Autodesk Inventor part; units mm, degrees
ref_plane "YZ Plane" through (0, 0, 0) normal (1, 0, 0) x (0, 1, 0)
ref_plane "XZ Plane" through (0, 0, 0) normal (0, 1, 0) x (-1, 0, 0)
ref_plane "XY Plane" through (0, 0, 0) normal (0, 0, 1) x (1, 0, 0)
sketch "Sketch1" plane through (0, 0, 0) normal (0, 1, 0) x (-1, 0, 0)
  circle A0 centre (0, 0) radius 10.16
  dimension "d0" = 20.32
extrude "Extrusion1" add sketch "Sketch1" along normal blind 31.75
sketch "Sketch2" plane through (0, 31.75, 0) normal (0, 1, 0) x (1, 0, 0)
  point P0 (0, 0)
  point P1 (0, 0)
hole "Hole1" at (0, 31.75, 0) direction (0, -1, 0) diameter 6.604 depth 19.05 tip angle 118
fillet "Fillet1" radius 3.175 1 edges at (10.16, 0, 0)
properties part number "legs"
Here's how the part is built. I have some questions about the finished solid (model axes, mm). Coordinates: 2 decimals unless noted, no trailing zeros. Order: outer loops, then holes, each group sorted by start corner. A loop starts at its lowest first (then second) coordinate and runs counter-clockwise, first axis right, second up. Notation, with made-up numbers: (-35, -24.75) - (-14, -24.75) arc R8 cw to (-14, -11.75) - close; hole circle Ø2 at (89.25, -33). An arc over 180 degrees is marked (long way). One line per question, with ' | ' between items. Start each with the question number.
1. I'm going to push flat-ended pins straight in: pin 1 Ø6 at (x, z) = (-5.5, 2) entering from -Y; pin 2 Ø2 at (x, y) = (-2.5, 15) entering from +Z; pin 3 Ø1.5 at (x, y) = (6, 21.5) entering from +Z; pin 4 Ø6 at (x, y) = (7, 21.5) entering from -Z. Where does each tip first touch, or does it pass through?
2. If we section it at A-A (y = 28): Write out the boundary of the cut face in (x, z), and give its area (3 significant figures).
3. If we mould it in two halves opening along Z, with no side actions, what happens to faces 1 (the cylindrical face through (1.323, 17.262, -10.074)), 2 (the cylindrical face through (1.26, 22.09, 3.05)), 3 (the flat face through (0, 0, 0))? For each: released by +Z, released by -Z, zero draft, split by the parting line, or undercut.
4. Please list where these lines run through material, in increasing order: line 1 along Z through (x, y) = (0, 21.5); line 2 along Y through (x, z) = (4, 8.5); line 3 along Y through (x, z) = (0.5, -8.25). Write a range as [from, to].
Model answer:
1) pin 1: stops at y = 0 | pin 2: stops at z = 10.05 | pin 3: stops at z = 8.7 | pin 4: stops at z = -9.34
2) outline: circle Ø20.32 at (0, 0); hole circle Ø6.6 at (0, 0) | area: 290 mm²
3) face 1: split by the parting line | face 2: undercut | face 3: zero draft
4) line 1: z = [-10.16, -3.3], [3.3, 10.16] | line 2: y = [1.11, 31.75] | line 3: y = [0.27, 31.75]
